Geometry check sheet. Reference: the model listing, model coordinates, mm. Round coordinates to 2 decimals unless told otherwise and drop trailing zeros. Write each loop counter-clockwise with the first axis right and the second up, starting at its lowest first coordinate (ties: lowest second). Pieces come first, ordered by that corner, then holes. Notation, with made-up numbers: (-18, 60.5) - (7, 60.5) arc R21 ccw to (7, 95.5) - close; hole circle Ø2 at (12, -25). An arc over 180 degrees is marked (long way). Return JSON: item names as keys, results as strings. Group by question number.
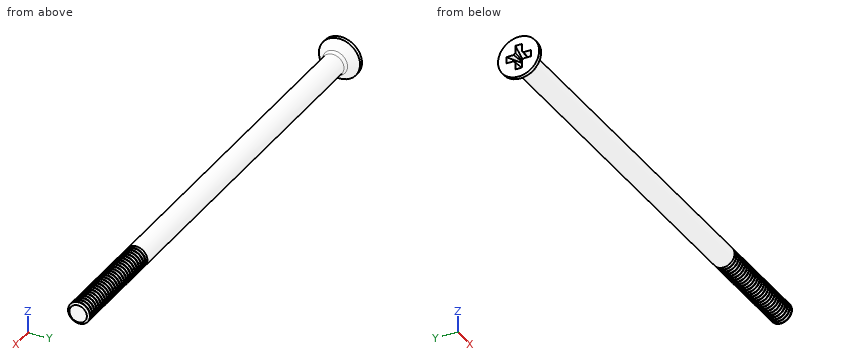
from build123d import *

# Parameters (mm, degrees)
FILLET1_R       = 0.6
RECPAT_COUNT    = 2
RECPAT_ANGLE    = 90
THDSCHPAT_COUNT = 28
THDSCHPAT_PITCH = 0.444444444


with BuildPart() as part:
    # BodySke → Base-Revolve (revolve)
    with BuildSketch(Plane.XY, mode=Mode.PRIVATE) as base_revolve_sk:
        Polygon((0, 0), (0, 2.35), (0.4, 2.35), (1.5, 1.25), (55, 1.25), (55, 0), align=None)
    revolve(base_revolve_sk.sketch.rotate(Axis((-6.35, 0, 0), (1, 0, 0)), 90), axis=Axis((-6.35, 0, 0), (1, 0, 0)))

    # Fillet1
    fillet1_edges = [part.edges().sort_by_distance(p)[0] for p in [
        (1.5, 0, -1.25),
    ]]
    fillet(fillet1_edges, radius=FILLET1_R)

    # Sketch3 → Recess section 0
    with BuildSketch(Plane.ZY):
        with BuildLine():
            Line((-0.37, 1.4), (0.37, 1.4))
            Line((0.37, 1.4), (0.37, -1.4))
            Line((0.37, -1.4), (-0.37, -1.4))
            Line((-0.37, -1.4), (-0.37, 1.4))
        make_face()
    # Sketch4 → Recess section 1
    with BuildSketch(Plane.ZY.offset(-1.73)):
        with BuildLine():
            Line((-0.37, 0.537453848), (0.37, 0.537453848))
            Line((0.37, 0.537453848), (0.37, -0.537453848))
            Line((0.37, -0.537453848), (-0.37, -0.537453848))
            Line((-0.37, -0.537453848), (-0.37, 0.537453848))
        make_face()
    recess = loft(mode=Mode.SUBTRACT)

    # RecPat: Recess ×2 about axis
    recpat_axis = Axis((0, 0, 0), (1, 0, 0))
    for i in range(1, RECPAT_COUNT):
        add(recess.rotate(recpat_axis, i * RECPAT_ANGLE / (RECPAT_COUNT - 1)), mode=Mode.SUBTRACT)

    # RecCorSke → RecessCore (revolve, cut)
    with BuildSketch(Plane.XY, mode=Mode.PRIVATE) as recesscore_sk:
        Polygon((0, 0), (0, 0.676973385), (1.73, 0.556), (1.910655351, 0), align=None)
    revolve(recesscore_sk.sketch.rotate(Axis((-3.175, 0, 0), (1, 0, 0)), 90), axis=Axis((-3.175, 0, 0), (1, 0, 0)), mode=Mode.SUBTRACT)

    # ThdSchSke → ThreadSchematic (revolve, cut)
    with BuildSketch(Plane.XY, mode=Mode.PRIVATE) as threadschematic_sk:
        Polygon((43.000001, -0.9965), (42.822498389, -1.25), (42.822498389, -1.5625), (43.177503611, -1.5625), (43.177503611, -1.25), align=None)
    threadschematic = revolve(threadschematic_sk.sketch.rotate(Axis((-3.175, 0, 0), (1, 0, 0)), 270), axis=Axis((-3.175, 0, 0), (1, 0, 0)), mode=Mode.SUBTRACT)

    # ThdSchPat: ThreadSchematic ×28
    with Locations(*[(i * THDSCHPAT_PITCH, 0, 0) for i in range(1, THDSCHPAT_COUNT)]):
        add(threadschematic, mode=Mode.SUBTRACT)


solid = part.part
1. Material ranges on line 1 along X through (y, z) = (-1.9, 1.05); line 2 along Z through (x, y) = (8.5, 0.15); line 3 along Z through (x, y) = (5, -0.65), recorded low to high.
2. Section check A-A (x = 40). Enter the section's corners in (y, z), and give its area (3 significant figures).
3. Depth check by flat-ended pin: pin 1 Ø1.5 at (x, z) = (27, 0.5) entering from -Y; pin 2 Ø1 at (x, y) = (39.5, 0) entering from +Z; pin 3 Ø2 at (x, z) = (47, 1) entering from +Y. Enter the tip coordinate at first touch or a pass-through.
Result sheet:
{
 "1": {"line 1": "x = 0 to 0.58", "line 2": "z = -1.24 to 1.24", "line 3": "z = -1.07 to 1.07"},
 "2": {"outline": "circle Ø2.5 at (0, 0)", "area": "4.91 mm²"},
 "3": {"pin 1": "stops at y = -1.25", "pin 2": "stops at z = 1.25", "pin 3": "stops at y = 1.25"}
}
